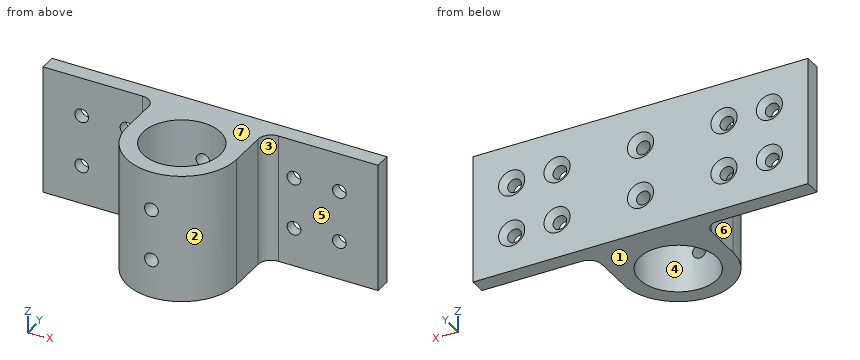
from build123d import *

# Parameters (mm, degrees)
BOSS_EXTRUDE1_DEPTH                                 = 31.75
SKETCH3_R                                           = 19.05
CUT_EXTRUDE1_DEPTH                                  = 64.5
CSK_FOR_1_4_FLAT_HEAD_MACHINE_SCREW_100_D           = 6.7564
CSK_FOR_1_4_FLAT_HEAD_MACHINE_SCREW_100_CSINK_D     = 12.8778
CSK_FOR_1_4_FLAT_HEAD_MACHINE_SCREW_100_CSINK_ANGLE = 100


with BuildPart() as part:
    # Sketch2 → Boss-Extrude1 (new body, symmetric)
    with BuildSketch(Plane.XY):
        with BuildLine():
            Line((82.55, 0), (-82.55, 0))
            Line((-82.55, 0), (-82.55, -7.9502))
            Line((-82.55, -7.9502), (-33.401, -7.9502))
            ThreePointArc((-33.401, -7.9502), (-28.910871939, -9.810071939), (-27.051, -14.3002))
            Line((-27.051, -14.3002), (-27.051, -33.3502))
            ThreePointArc((-27.051, -33.3502), (0, -60.4012), (27.051, -33.3502))
            Line((27.051, -33.3502), (27.051, -14.3002))
            ThreePointArc((27.051, -14.3002), (28.910871939, -9.810071939), (33.401, -7.9502))
            Line((33.401, -7.9502), (82.55, -7.9502))
            Line((82.55, -7.9502), (82.55, 0))
        make_face()
    extrude(amount=BOSS_EXTRUDE1_DEPTH, both=True)

    # Sketch3 → Cut-Extrude1 (cut, through all)
    with BuildSketch(Plane.XY.offset(31.75)):
        with Locations((0, -33.3502)):
            Circle(SKETCH3_R)
    extrude(amount=-CUT_EXTRUDE1_DEPTH, mode=Mode.SUBTRACT)

    # CSK for 1/4 Flat Head Machine Screw (100)2 (through all)
    with Locations(Plane(origin=(0, 0, 0), x_dir=(1, 0, 0), z_dir=(0, 1, 0))):
        with Locations((0, -12.7), (41.148, -12.7), (63.5, -12.7), (-41.148, -12.7), (-63.5, -12.7), (-41.148, 12.7), (-63.5, 12.7), (0, 12.7), (41.148, 12.7), (63.5, 12.7)):
            CounterSinkHole(CSK_FOR_1_4_FLAT_HEAD_MACHINE_SCREW_100_D / 2, CSK_FOR_1_4_FLAT_HEAD_MACHINE_SCREW_100_CSINK_D / 2, counter_sink_angle=CSK_FOR_1_4_FLAT_HEAD_MACHINE_SCREW_100_CSINK_ANGLE)


solid = part.part
Geometry: final body of the model. Coordinates: model frame, mm. Face numbers are marked on the shaded views. A direction names the side the tool comes from. Round coordinates to 2 decimals unless told otherwise and drop trailing zeros. Loops run counter-clockwise (first coordinate to the right, second up) from the corner with the lowest first, then second, coordinate; pieces in that order, holes last. Notation, with made-up numbers: M -7.75,8 L 12.25,8 A7 ccw 12.25,17 Z; hole C -7,71 d3. An arc over 180 degrees is marked long. One line per question, with ' | ' between items.
(1) Contact query for flat-ended pins moving along their axis: P1, Ø8, axis at y = -22.5, z = 16.5, coming from the +X side; P2, Ø3, axis at y = -10, z = 23, coming from the +X side; P3, Ø9, axis at x = -41.148, z = -12.7, coming from the -Y side. Output: stop coordinate, or through.
Check result:
P1: stops at x = 27.05 | P2: stops at x = 30.82 | P3: stops at y = -7.95
(2) Access query for the marked faces 5, 6 and 7. Directions: +Z, -Z, +X, -X, +Y, -Y. A direction counts if a zero-diameter tool reaches every point of the face in a straight line with its end or side. Return the directions, or none.
Check result:
face 5: +Z, -Z, +X, -Y | face 6: +Z, -Z, -X, -Y | face 7: +Z, +X, -X, +Y, -Y
(3) Pull-direction query (X, two-part tool) for the marked faces 1, 2, 3 and 4; classes: +X half, -X half, draft (parallel to the pull), parting line (faces both ways), or undercut.
Check result:
face 1: draft | face 2: parting line | face 3: +X half | face 4: undercut
(4) Material intervals for line 1 along Z through (x, y) = (0, -57); line 2 along Z through (x, y) = (63, -4); line 3 along X through (y, z) = (-4.6, -12.7), sorted ascending. Write a range as from..to.
Check result:
line 1: z = -31.75..-16.08, -9.32..9.32, 16.08..31.75 | line 2: z = -31.75..-16.04, -9.36..9.36, 16.04..31.75 | line 3: x = -82.55..-66.88, -60.12..-44.53, -37.77..-3.38, 3.38..37.77, 44.53..60.12, 66.88..82.55
(5) Cut plane C-C on x = -63.5. Return the cut outline in (y, z), plus the area to 3 significant figures.
Check result:
outline: M -7.95,-31.75 L 0,-31.75 L 0,-19.14 L -2.57,-16.08 L -7.95,-16.08 Z; M -7.95,-9.32 L -2.57,-9.32 L 0,-6.26 L 0,6.26 L -2.57,9.32 L -7.95,9.32 Z; M -7.95,16.08 L -2.57,16.08 L 0,19.14 L 0,31.75 L -7.95,31.75 Z | area: 382 mm2
(6) Cut plane B-B on y = -17. Return the cut outline in (x, z), plus the area to 3 significant figures.
Check result:
outline: M -27.05,-31.75 L -9.78,-31.75 L -9.78,31.75 L -27.05,31.75 Z; M 9.78,-31.75 L 27.05,-31.75 L 27.05,31.75 L 9.78,31.75 Z | area: 2,190 mm2
(7) Cut plane D-D on y = -50.5. Return the cut outline in (x, z).
Check result:
outline: M -20.92,-31.75 L -8.29,-31.75 L -8.29,31.75 L -20.92,31.75 Z; M 8.29,-31.75 L 20.92,-31.75 L 20.92,31.75 L 8.29,31.75 Z
(8) Cut plane A-A on z = 2.5. Return the cut outline in (x, y), plus the area to 3 significant figures.
Check result:
outline: M -82.55,-7.95 L -33.4,-7.95 A6.35 cw -27.05,-14.3 L -27.05,-33.35 A27.05 ccw 27.05,-33.35 L 27.05,-14.3 A6.35 cw 33.4,-7.95 L 82.55,-7.95 L 82.55,0 L -82.55,0 Z; hole C 0,-33.35 d38.1 | area: 2,710 mm2
